from build123d import *

# Parameters (mm, degrees)
CROQUIS1_R              = 8
SALIENTE_EXTRUIR1_DEPTH = 10
SALIENTE_EXTRUIR2_DEPTH = 10
CROQUIS3_R              = 11
CORTAR_EXTRUIR1_DEPTH   = 122.2930336


with BuildPart() as part:
    # Croquis1 → Saliente-Extruir1 (new body)
    with BuildSketch(Plane.XY):
        with BuildLine():
            Line((-32.224593289, 23.697586108), (-69.917911477, -27.558767293))
            ThreePointArc((-69.917911477, -27.558767293), (-73.915346544, -38.116312412), (-71.868614208, -49.218210124))
            Line((-71.868614208, -49.218210124), (-54.376087015, -85.023398189))
            ThreePointArc((-54.376087015, -85.023398189), (-36.395654862, -93.588736194), (-24, -78))
            ThreePointArc((-24, -78), (0, -54), (24, -78))
            ThreePointArc((24, -78), (36.395654862, -93.588736194), (54.376087015, -85.023398189))
            Line((54.376087015, -85.023398189), (71.868614208, -49.218210124))
            ThreePointArc((71.868614208, -49.218210124), (73.915346544, -38.116312412), (69.917911477, -27.558767293))
            Line((69.917911477, -27.558767293), (32.224593289, 23.697586108))
            ThreePointArc((32.224593289, 23.697586108), (0, 40), (-32.224593289, 23.697586108))
        make_face()
        with Locations((-40, -78)):
            Circle(CROQUIS1_R, mode=Mode.SUBTRACT)
        with Locations((40, -78)):
            Circle(CROQUIS1_R, mode=Mode.SUBTRACT)
    extrude(amount=SALIENTE_EXTRUIR1_DEPTH)

    # Croquis2 → Saliente-Extruir2 (add)
    with BuildSketch(Plane.XY.offset(10)):
        with BuildLine():
            ThreePointArc((32.224593289, 23.697586108), (0, 40), (-32.224593289, 23.697586108))
            ThreePointArc((-32.224593289, 23.697586108), (-12.470290061, -38.006471367), (40, 0))
            ThreePointArc((40, 0), (38.006471367, 12.470290061), (32.224593289, 23.697586108))
        make_face()
        with BuildLine():
            ThreePointArc((-32, -40), (-46.453097718, -20.046602532), (-69.917911477, -27.558767293))
            ThreePointArc((-69.917911477, -27.558767293), (-73.915346544, -38.116312412), (-71.868614208, -49.218210124))
            ThreePointArc((-71.868614208, -49.218210124), (-48.269297006, -60.460216254), (-32, -40))
        make_face()
        with BuildLine():
            ThreePointArc((74, -40), (72.953397468, -33.453097718), (69.917911477, -27.558767293))
            ThreePointArc((69.917911477, -27.558767293), (32.084653456, -41.883687588), (71.868614208, -49.218210124))
            ThreePointArc((71.868614208, -49.218210124), (73.460216254, -44.730702994), (74, -40))
        make_face()
    extrude(amount=SALIENTE_EXTRUIR2_DEPTH)

    # Croquis3 → Cortar-Extruir1 (cut, through all)
    with BuildSketch(Plane.XY.offset(20)):
        with BuildLine():
            Line((-12.410406251, -29.49545417), (-6.843662449, -19.853571071))
            ThreePointArc((-6.843662449, -19.853571071), (0, -21), (6.843662449, -19.853571071))
            Line((6.843662449, -19.853571071), (12.410406251, -29.49545417))
            Line((12.410406251, -29.49545417), (19.338609482, -25.49545417))
            Line((19.338609482, -25.49545417), (13.771865679, -15.853571071))
            ThreePointArc((13.771865679, -15.853571071), (18.186533479, -10.5), (20.615528128, -4))
            Line((20.615528128, -4), (31.749015733, -4))
            Line((31.749015733, -4), (31.749015733, 4))
            Line((31.749015733, 4), (20.615528128, 4))
            ThreePointArc((20.615528128, 4), (18.186533479, 10.5), (13.771865679, 15.853571071))
            Line((13.771865679, 15.853571071), (19.338609482, 25.49545417))
            Line((19.338609482, 25.49545417), (12.410406251, 29.49545417))
            Line((12.410406251, 29.49545417), (6.843662449, 19.853571071))
            ThreePointArc((6.843662449, 19.853571071), (0, 21), (-6.843662449, 19.853571071))
            Line((-6.843662449, 19.853571071), (-12.410406251, 29.49545417))
            Line((-12.410406251, 29.49545417), (-19.338609482, 25.49545417))
            Line((-19.338609482, 25.49545417), (-13.771865679, 15.853571071))
            ThreePointArc((-13.771865679, 15.853571071), (-18.186533479, 10.5), (-20.615528128, 4))
            Line((-20.615528128, 4), (-31.749015733, 4))
            Line((-31.749015733, 4), (-31.749015733, -4))
            Line((-31.749015733, -4), (-20.615528128, -4))
            ThreePointArc((-20.615528128, -4), (-18.186533479, -10.5), (-13.771865679, -15.853571071))
            Line((-13.771865679, -15.853571071), (-19.338609482, -25.49545417))
            Line((-19.338609482, -25.49545417), (-12.410406251, -29.49545417))
        make_face()
        with Locations((53, -40)):
            Circle(CROQUIS3_R)
        with Locations((-53, -40)):
            Circle(CROQUIS3_R)
    extrude(amount=-CORTAR_EXTRUIR1_DEPTH, mode=Mode.SUBTRACT)


solid = part.part
Can you work these out from the model? Positions are in its coordinate system, mm. A direction names the side the tool comes from. Give positions to 0.01 mm unless a question says otherwise; leave off trailing zeros. Order: outer loops, then holes, each group sorted by start corner. A loop starts at its lowest first (then second) coordinate and runs counter-clockwise, first axis right, second up. Notation, with made-up numbers: M 51,-7.5 L 93,-7.5 A16 ccw 93,-0.5 Z; hole C 75,89.25 d3. An arc over 180 degrees is marked long. One line per question, with ' | ' between items.
Item 1: Suppose I cut it at C-C, the plane y = 7.5. Write out the boundary of the cut face in (x, z), then the cut area to 3 significant figures.
Answer block:
outline: M -44.14,0 L -19.62,0 L -19.62,20 L -39.29,20 L -39.29,10 L -44.14,10 Z; M 19.62,0 L 44.14,0 L 44.14,10 L 39.29,10 L 39.29,20 L 19.62,20 Z | area: 884 mm2
Item 2: We'd pull the mould along Y, two halves only. Please class faces 4 (the face through (26, -4, 10)), 5 (the face through (-1, -26, 0)), 6 (the face through (-0.528, -54.006, 4.93)), 7 (the face through (51.335, -2.289, 4.93)): released by +Y, released by -Y, zero draft, split by the parting line, or undercut.
Answer block:
face 4: undercut | face 5: zero draft | face 6: released by -Y | face 7: released by +Y
Item 3: Please list where these lines run through material, in increasing order: L1, parallel to Y at x = -16, z = 11.25; L2, parallel to X at y = -35, z = 4.5; L3, parallel to Z at x = -50.5, y = -61.
Answer block:
L1: y = -36.66 to -27.42, -19.71 to -13.6, 13.6 to 19.71, 27.42 to 36.66 | L2: x = -73.4 to -62.8, -43.2 to 43.2, 62.8 to 73.4 | L3: z = 0 to 10
Item 4: Suppose I cut it at D-D, the plane y = -82.5. Write out the boundary of the cut face in (x, z).
Answer block:
outline: M -55.61,0 L -46.61,0 L -46.61,10 L -55.61,10 Z; M -33.39,0 L -24.65,0 L -24.65,10 L -33.39,10 Z; M 24.65,0 L 33.39,0 L 33.39,10 L 24.65,10 Z; M 46.61,0 L 55.61,0 L 55.61,10 L 46.61,10 Z
Item 5: Suppose I cut it at B-B, the plane z = 13.5. Give the number of separate pieces and of enclosed holes in the cut face, then the cut area to 3 significant figures.
Answer block:
separate pieces: 3 | enclosed holes: 3 | area: 5,130 mm2
Item 6: For faces 1 (the face through (0, 21, 10)), 2 (the face through (-44, -49, 20)), 3 (the face through (0, -52, 10)), which set-ups out of +Z, -Z, +X, -X, +Y, -Y let a thin tool reach every point of the face, with its end or its side?
Answer block:
face 1: +Z, -Z | face 2: +Z, +X, -X, +Y, -Y | face 3: +Z
Item 7: I'm going to push flat-ended pins straight in: pin 1 Ø8 at (y, z) = (-11.5, 5) entering from -X; pin 2 Ø13 at (x, y) = (53, -40) entering from +Z; pin 3 Ø10 at (y, z) = (-12, 3) entering from +X; pin 4 Ø12 at (x, z) = (25, 7) entering from -Y. Where does each tip first touch, or does it pass through?
Answer block:
pin 1: stops at x = -61.05 | pin 2: passes through | pin 3: stops at x = 62.15 | pin 4: stops at y = -91.23
Item 8: Suppose I cut it at A-A, the plane x = 0. Write out the boundary of the cut face in (y, z), then the cut area to 3 significant figures.
Answer block:
outline: M -54,0 L -21,0 L -21,20 L -40,20 L -40,10 L -54,10 Z; M 21,0 L 40,0 L 40,20 L 21,20 Z | area: 900 mm2
